from build123d import *

# Parameters (mm, degrees)
EXTRUDE_1_DEPTH     = 6.5
CUT_EXTRUDE_1_DEPTH = 52.886896226
CUT_EXTRUDE_2_DEPTH = 54.09425581


with BuildPart() as part:
    # 草图1 → 凸台-拉伸1 (new, symmetric)
    with BuildSketch(Plane.XY):
        with BuildLine():
            Line((0, 0), (0, 6))
            ThreePointArc((0, 6), (5.87927664, 28.388613177), (22, 45))
            Line((22, 45), (25, 45))
            Line((25, 45), (25, 42))
            ThreePointArc((25, 42), (21.416586692, 24), (25, 6))
            Line((25, 6), (20, 6))
            Line((20, 6), (20, 0))
            Line((20, 0), (0, 0))
        make_face()
    extrude(amount=EXTRUDE_1_DEPTH, both=True)

    # 草图2 → 切除-拉伸1 (cut, through all)
    with BuildSketch(Plane.ZY):
        Polygon((6.5, 4.253461365), (3.25, 4.253461365), (4, 0), (6.5, 0), align=None)
        Polygon((-4, 0), (-6.5, 0), (-6.5, 4.253461365), (-3.25, 4.253461365), align=None)
    extrude(amount=-CUT_EXTRUDE_1_DEPTH, mode=Mode.SUBTRACT)

    # 草图3 → 切除-拉伸2 (cut, through all)
    with BuildSketch(Plane.XY.offset(6.5)):
        with BuildLine():
            ThreePointArc((6.932463861, 12.026105414), (12.037858369, 12.649666202), (17.162813582, 12.215252555))
            ThreePointArc((17.162813582, 12.215252555), (19.038256161, 12.860028298), (19.436438993, 14.802828097))
            ThreePointArc((19.436438993, 14.802828097), (17.311240055, 24.38211379), (17.097768587, 34.191987125))
            ThreePointArc((17.097768587, 34.191987125), (15.842511021, 36.203388469), (13.548853711, 35.602936079))
            ThreePointArc((13.548853711, 35.602936079), (7.517605312, 25.546939135), (4.501465211, 14.215481563))
            ThreePointArc((4.501465211, 14.215481563), (5.148632601, 12.489739676), (6.932463861, 12.026105414))
        make_face()
    extrude(amount=-CUT_EXTRUDE_2_DEPTH, mode=Mode.SUBTRACT)


solid = part.part
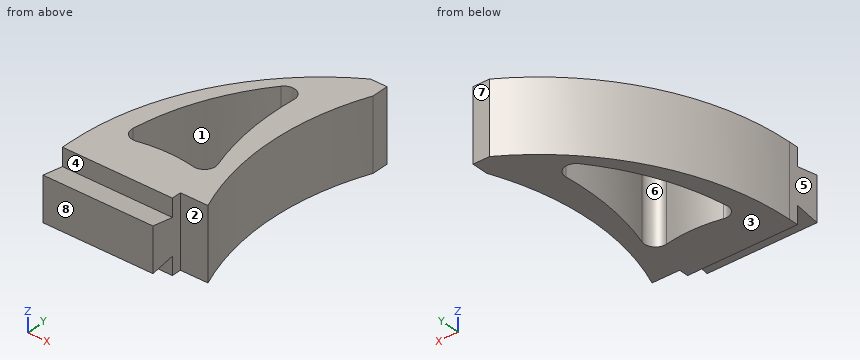
Input: part model. Units: mm. Frame: model coordinates. Face numbers are marked on the shaded views. A direction names the side the tool comes from. Give positions to 0.01 mm unless a question says otherwise; leave off trailing zeros. Loops run counter-clockwise (first coordinate to the right, second up) from the corner with the lowest first, then second, coordinate; pieces in that order, holes last. Notation, with made-up numbers: (84.5, 88.5) - (95.5, 88.5) arc R25 ccw to (95.5, 126.5) - close; hole circle Ø8 at (75, 47.5). An arc over 180 degrees is marked (long way). Use CSV: the item, a comma, the result in double quotes. Start each with the question number.
Item 1: Mould query, pull axis Y, two halves, no side actions, for the marked faces 6, 7 and 8. Classes: pulls with the +Y half, pulls with the -Y half, needs draft (parallel to the pull), parting line crosses it, or undercut.
Item 2: Reachability of the marked faces 1, 2, 3, 4 and 5 from +Z, -Z, +X, -X, +Y, -Y: full face, straight path, thin tool, end or side. Return the list, or none.
Item 3: Section D-D on x = 3.75. Return loops of the section in (y, z), then the cut area to 3 significant figures.
Item 4: Section B-B on z = 0.75. Return loops of the section in (x, y), then the cut area to 3 significant figures.
Item 5: Contact query for flat-ended pins moving along their axis: P1, Ø2, axis at y = 11.5, z = -2, coming from the +X side; P2, Ø1, axis at y = 36.5, z = 4, coming from the -X side. Output: stop coordinate, or through.
Item 6: Section A-A on x = 18.75. Return loops of the section in (y, z), then the cut area to 3 significant figures.
Item 7: Section C-C on y = 32.5. Return loops of the section in (x, z), then the cut area to 3 significant figures.
Item 8: Line query: line 1 (X direction, y = 19.5, z = 1.75); line 2 (X direction, y = 20.5, z = 3); line 3 (X direction, y = 5.5, z = 2). Output: solid intervals per line, ascending.
Ans:
1,face 6,"undercut"
1,face 7,"pulls with the +Y half"
1,face 8,"pulls with the -Y half"
2,face 1,"+Z, -Z"
2,face 2,"+Z, -Z, +X, -Y"
2,face 3,"-Z, +X, -X, +Y, -Y"
2,face 4,"+Z, +X, -X"
2,face 5,"+Z, -Z, -X, +Y, -Y"
3,outline,"(0, -4) - (4.25, -3.25) - (4.25, -6.5) - (24.1, -6.5) - (24.1, 6.5) - (4.25, 6.5) - (4.25, 3.25) - (0, 4) - close"
3,area,"289 mm2"
4,outline,"(0, 0) - (20, 0) - (20, 6) - (25, 6) arc R47 cw to (25, 42) - (25, 45) - (22, 45) arc R45.57 ccw to (0, 6) - close; hole (4.5, 14.22) arc R2 ccw to (6.93, 12.03) arc R25 cw to (17.16, 12.22) arc R2 ccw to (19.44, 14.8) arc R50 cw to (17.1, 34.19) arc R2 ccw to (13.55, 35.6) arc R42 ccw to start"
4,area,"520 mm2"
5,P1,"stops at x = 23.4"
5,P2,"stops at x = 11.27"
6,outline,"(0, -4) - (4.25, -3.25) - (4.25, -6.5) - (12.59, -6.5) - (12.59, 6.5) - (4.25, 6.5) - (4.25, 3.25) - (0, 4) - close; (17.08, -6.5) - (42.84, -6.5) - (42.84, 6.5) - (17.08, 6.5) - close"
6,area,"474 mm2"
7,outline,"(8.5, -6.5) - (11.27, -6.5) - (11.27, 6.5) - (8.5, 6.5) - close; (17, -6.5) - (22.19, -6.5) - (22.19, 6.5) - (17, 6.5) - close"
7,area,"104 mm2"
8,line 1,"x = 2.05 to 5.49, 18.15 to 21.63"
8,line 2,"x = 2.37 to 5.75, 17.94 to 21.55"
8,line 3,"x = 0 to 20"
